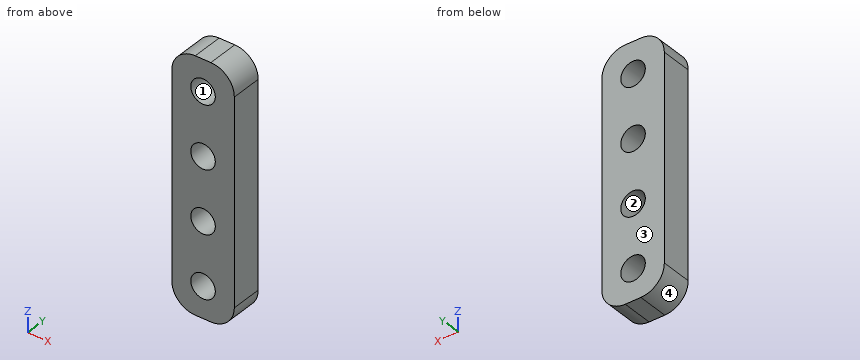
```python
from build123d import *

# Parameters (mm, degrees)
SKETCH1_W           = 12.7
SKETCH1_H           = 50.8
SKETCH1_R           = 2.4892
BOSS_EXTRUDE1_DEPTH = 6.35
LPATTERN1_OUTLINE_R = 2.4892
LPATTERN1_DEPTH     = 6.35
FILLET1_R           = 4.7625


# Read off the part's stored shape, not the designer's step: LPattern1
with BuildPart() as part:
    # Sketch1 → Boss-Extrude1 (new body)
    with BuildSketch(Plane(origin=(0, 0, 0), x_dir=(1, 0, 0), z_dir=(0, 1, 0))):
        with Locations((6.35, 25.4)):
            Rectangle(SKETCH1_W, SKETCH1_H)
        with Locations(Location((6.35, 6.35, 0), (0, 0, 270))):
            Circle(SKETCH1_R, mode=Mode.SUBTRACT)
    extrude(amount=BOSS_EXTRUDE1_DEPTH)

    # LPattern1 outline → LPattern1 (cut)
    with BuildSketch(Plane(origin=(0, 0, 0), x_dir=(1, 0, 0), z_dir=(0, 1, 0))):
        with Locations((6.35, 44.45)):
            Circle(LPATTERN1_OUTLINE_R)
        with Locations((6.35, 31.75)):
            Circle(LPATTERN1_OUTLINE_R)
        with Locations((6.35, 19.05)):
            Circle(LPATTERN1_OUTLINE_R)
    extrude(amount=LPATTERN1_DEPTH, mode=Mode.SUBTRACT)

    # Fillet1
    fillet1_edges = [part.edges().sort_by_distance(p)[0] for p in [
        (0, 3.175, -50.8),
        (12.7, 3.175, -50.8),
        (12.7, 3.175, 0),
        (0, 3.175, 0),
    ]]
    fillet(fillet1_edges, radius=FILLET1_R)


solid = part.part
```
Model file for the job. Use its own axes, mm. Face numbers are marked on the shaded views. Coordinates: 2 decimals unless noted, no trailing zeros. Loops run counter-clockwise (first coordinate to the right, second up) from the corner with the lowest first, then second, coordinate; pieces in that order, holes last. Notation, with made-up numbers: (-36, 5.25) -> (-4, 5.25) arc R18 cw to (-4, 32.25) -> close; hole circle Ø1 at (5, 4.25). An arc over 180 degrees is marked (long way). Answer as a JSON object with one key per item and string values.
Q1. Cut at A-A (x = 6.35). List the corners of the cut face in (y, z), and give its area (3 significant figures).
Report:
{"outline": "(0, -50.8) -> (6.35, -50.8) -> (6.35, -46.94) -> (0, -46.94) -> close; (0, -41.96) -> (6.35, -41.96) -> (6.35, -34.24) -> (0, -34.24) -> close; (0, -29.26) -> (6.35, -29.26) -> (6.35, -21.54) -> (0, -21.54) -> close; (0, -16.56) -> (6.35, -16.56) -> (6.35, -8.84) -> (0, -8.84) -> close; (0, -3.86) -> (6.35, -3.86) -> (6.35, 0) -> (0, 0) -> close", "area": "196 mm2"}
Q2. Probe probe 1 along X at (y, z) = (1.5, -19.05); probe 2 along Z at (x, y) = (5.75, 1.25); probe 3 along Z at (x, y) = (11.25, 5). List the from-to ranges inside material, lowest first.
Report:
{"probe 1": "x = 0 to 3.86, 8.84 to 12.7", "probe 2": "z = -50.8 to -46.87, -42.03 to -34.17, -29.33 to -21.47, -16.63 to -8.77, -3.93 to 0", "probe 3": "z = -49.46 to -1.34"}
Q3. Cut at D-D (z = -31.75). List the corners of the cut face in (x, y).
Report:
{"outline": "(0, 0) -> (3.86, 0) -> (3.86, 6.35) -> (0, 6.35) -> close; (8.84, 0) -> (12.7, 0) -> (12.7, 6.35) -> (8.84, 6.35) -> close"}
Q4. Cut at B-B (z = -5.5). List the corners of the cut face in (x, y).
Report:
{"outline": "(0, 0) -> (4.01, 0) -> (4.01, 6.35) -> (0, 6.35) -> close; (8.69, 0) -> (12.7, 0) -> (12.7, 6.35) -> (8.69, 6.35) -> close"}
Q5. Cut at C-C (y = 2). State how many separate pieces and enclosed holes the cut face has, and give its area (3 significant figures).
Report:
{"separate pieces": "1", "enclosed holes": "4", "area": "548 mm2"}
Q6. Pull direction Z, two halves, no side cores. Call the marked faces 1, 2, 3 and 4: released by +Z, released by -Z, zero draft, split by the parting line, or undercut.
Report:
{"face 1": "undercut", "face 2": "undercut", "face 3": "zero draft", "face 4": "released by -Z"}
